Model file for the job. Use its own axes, mm. Round coordinates to 2 decimals unless told otherwise and drop trailing zeros. Loops run counter-clockwise (first coordinate to the right, second up) from the corner with the lowest first, then second, coordinate; pieces in that order, holes last. Notation, with made-up numbers: M -22.5,50.5 L 16.5,50.5 A37 ccw 16.5,89.5 Z; hole C 36.5,24.5 d9. An arc over 180 degrees is marked long. Use a Markdown table: item, result. Add a question column.
Item 1: Saw through at D-D on y = -58.5. Write the cut outline in (x, z).
Item 2: Two-plate mould, pull along Y, no slides. Class faces 1 (the flat face through (1.5, -2, 118)), 2 (the flat face through (0, -74, 152)), 3 (the flat face through (0, 74, 152)): +Y half, -Y half, draft (parallel to the pull), parting line (faces both ways), or undercut.
Item 3: Saw through at C-C on z = 27. Write the cut outline in (x, y), then the cut area to 3 significant figures.
Item 4: Pin check, flat tips, straight feed: P1, Ø1.5, axis at x = 0.5, z = 45, coming from the +Y side (3 decimals); P2, Ø0.9, axis at x = 0, y = -0.5, coming from the -Z side; P3, Ø1, axis at x = 0, y = -75, coming from the +Z side. Stop position of each tip, or through.
Item 5: Saw through at B-B on x = -0.1. Write the cut outline in (y, z), then the cut area to 3 significant figures.
Item 6: Saw through at A-A on z = 70.5. Write the cut outline in (x, y).
Item 7: Wall check: L1, parallel to Y at x = 0.15, z = 45; L2, parallel to Y at x = 0.65, z = 44; L3, parallel to Y at x = -1, z = 164.5. Give the ranges that are in metal, low to high. Write a range as from..to.
Autodesk Inventor part; units mm, degrees
ref_plane "YZ Plane" through (0, 0, 0) normal (1, 0, 0) x (0, 1, 0)
ref_plane "XZ Plane" through (0, 0, 0) normal (0, 1, 0) x (-1, 0, 0)
ref_plane "XY Plane" through (0, 0, 0) normal (0, 0, 1) x (1, 0, 0)
sketch "Sketch1" plane through (0, 0, 0) normal (1, 0, 0) x (0, 1, 0)
  line L0 (150, 0) -> (-150, 0)
  line L1 (0, 0) -> (0, 300)
  line L2 (0, 300) -> (150, 0)
  line L3 (0, 300) -> (-150, 0)
  dimension "d0" = 300
  dimension "d1" = 300
extrude "Plate1" add sketch "Sketch1" along normal mid plane 3
sketch "Sketch3" plane through (1.5, 0, 0) normal (1, 0, 0) x (0, 0, -1)
  line L0 (0, -1.6) -> (-151, -1.6)
  line L1 (-151, -1.6) -> (-151, 1.6)
  line L2 (-151, 1.6) -> (0, 1.6)
  line L3 (0, 1.6) -> (0, -1.6)
  line L4 (0, 150) -> (0, -150)
  point P0 (0, 0)
  point P1 (0, 0)
  dimension "d7" = 3.2
  dimension "d8" = 151
extrude "Extrusion2" cut sketch "Sketch3" against normal through all
chamfer "Corner Chamfer1" distance 2 angle 45 1 edges at (0, 0, 300)
chamfer "Corner Chamfer2" distance 2 angle 45 2 edges at (0, -150, 0) (0, 150, 0)
equation "\"d2\" = Thickness"
equation "\"BendReliefWidth\" = Thickness"
equation "\"BendReliefDepth\" = 0.5 * Thickness"
equation "\"CornerReliefSize\" = 4 * Thickness"
equation "\"MinimumRemnant\" = 2 * Thickness"
equation "\"TransitionRadius\" = BendRadius"
equation "\"JacobiRadiusSize\" = BendRadius"
equation "\"GapSize\" = Thickness"
properties part number "MSC 207 CONE BLADE" material "Stainless Steel"
Entries:
| question | item | result |
|---|---|---|
| 1 | outline | M -1.5,0 L 1.5,0 L 1.5,183 L -1.5,183 Z |
| 2 | face 1 | draft |
| 2 | face 2 | -Y half |
| 2 | face 3 | +Y half |
| 3 | outline | M -1.5,-136.5 L 1.5,-136.5 L 1.5,-1.6 L -1.5,-1.6 Z; M -1.5,1.6 L 1.5,1.6 L 1.5,136.5 L -1.5,136.5 Z |
| 3 | area | 809 mm2 |
| 4 | P1 | y = 127.875 |
| 4 | P2 | z = 151 |
| 4 | P3 | z = 151 |
| 5 | outline | M -149.11,1.79 L -148,0 L -1.6,0 L -1.6,151 L 1.6,151 L 1.6,0 L 148,0 L 149.11,1.79 L 0.89,298.21 L -0.89,298.21 Z |
| 5 | area | 44,500 mm2 |
| 6 | outline | M -1.5,-114.75 L 1.5,-114.75 L 1.5,-1.6 L -1.5,-1.6 Z; M -1.5,1.6 L 1.5,1.6 L 1.5,114.75 L -1.5,114.75 Z |
| 7 | L1 | -127.5..-1.6, 1.6..127.5 |
| 7 | L2 | -128..-1.6, 1.6..128 |
| 7 | L3 | -67.75..67.75 |
